Study the drawing (mm; zero at the part's minimum x, y, z) and answer. A direction names the side the tool comes from. Round coordinates to 2 decimals unless told otherwise and drop trailing zeros. Write each loop counter-clockwise with the first axis right and the second up, starting at its lowest first coordinate (ties: lowest second). Pieces come first, ordered by that corner, then holes. Notation, with made-up numbers: (5, 66) - (51, 66) arc R23 cw to (51, 81) - close; hole circle Ø7 at (-4.5, 80.5). An arc over 180 degrees is marked (long way). Return JSON: item names as keys, results as strings. Group by question number.
(1) Section C-C, the plane y = 3 is taken. Write down the section's boundary in (x, z).
(2) Section B-B, the plane z = 4.4 is taken. Write down the section's boundary in (x, y) (1 decimal).
(3) Each of these flat-tipped pins is pushed along its axis until it touches: pin 1 (2 mm diameter, centred on x = 23, z = 4, fed in from -Y); pin 2 (1.4 mm diameter, centred on y = 12, z = 2, fed in from +X); pin 3 (5 mm diameter, centred on y = 2, z = 5.5, fed in from -X); pin 4 (4 mm diameter, centred on x = 181.41, z = 4.4, fed in from +Y). Where does it stop, or does it pass through?
(4) Find the intervals of material crossed by line 1 along Y through (x, z) = (142.5, 1.25) (1 decimal); line 2 along Z through (x, y) = (36.5, 19); line 3 along X through (y, z) = (5, 8.5), in increasing order. Write a range as [from, to].
(5) Section D-D, the plane x = 41.5 is taken. Write down the section's boundary in (y, z).
(6) Section A-A, the plane x = 146.5 is taken. Write down the section's boundary in (y, z) (1 decimal).
(7) Which of the six approach directions +Z, -Z, +X, -X, +Y, -Y give full straight-line access (tool end or side, diameter ignored) to the marked faces 1 and 2?
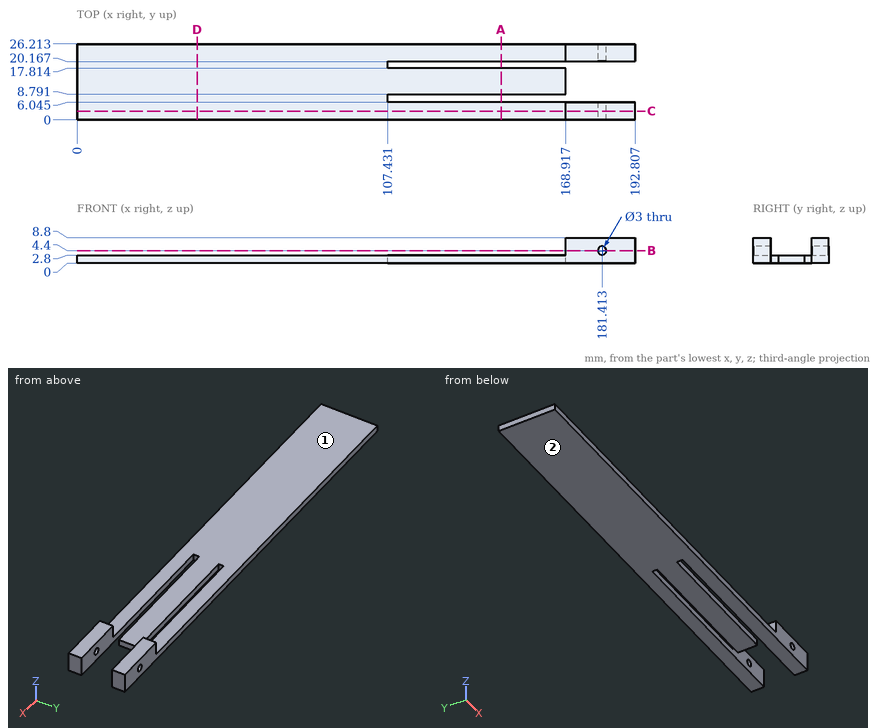
Working result:
{
 "1": {"outline": "(0, 0) - (192.81, 0) - (192.81, 8.8) - (168.92, 8.8) - (168.92, 2.8) - (0, 2.8) - close; hole circle Ø3 at (181.41, 4.4)"},
 "2": {"outline": "(168.9, 0) - (179.9, 0) - (179.9, 6) - (168.9, 6) - close; (168.9, 20.2) - (179.9, 20.2) - (179.9, 26.2) - (168.9, 26.2) - close; (182.9, 0) - (192.8, 0) - (192.8, 6) - (182.9, 6) - close; (182.9, 20.2) - (192.8, 20.2) - (192.8, 26.2) - (182.9, 26.2) - close"},
 "3": {"pin 1": "passes through", "pin 2": "stops at x = 168.92", "pin 3": "stops at x = 168.92", "pin 4": "stops at y = 26.21"},
 "4": {"line 1": "y = [0, 6], [8.8, 17.8], [20.2, 26.2]", "line 2": "z = [0, 2.8]", "line 3": "x = [168.92, 192.81]"},
 "5": {"outline": "(0, 0) - (26.21, 0) - (26.21, 2.8) - (0, 2.8) - close"},
 "6": {"outline": "(0, 0) - (6, 0) - (6, 2.8) - (0, 2.8) - close; (8.8, 0) - (17.8, 0) - (17.8, 2.8) - (8.8, 2.8) - close; (20.2, 0) - (26.2, 0) - (26.2, 2.8) - (20.2, 2.8) - close"},
 "7": {"face 1": "+Z, -X, +Y, -Y", "face 2": "-Z, +X, -X, +Y, -Y"}
}
